```python
from build123d import *

# Parameters (mm, degrees)
F0_W      = 92
F0_H      = 42.9992415011
F0_W_2    = 39.8767858334
F0_H_2    = 7.2647114284
F0_W_3    = 8.2464283332
F0_H_3    = 15.8676442858
F1_DEPTH  = 2
F2_W      = 8.2464283332
F2_H      = 1.5
F3_DEPTH  = 17
F4_DEPTH  = 17
F6_DEPTH  = 2
F7_W      = 8
F7_H      = 3
F8_DEPTH  = 1
F10_W     = 8
F10_H     = 8
F11_DEPTH = 1
F9_W      = 8
F9_H      = 8
F12_DEPTH = 1
F13_W     = 8
F13_H     = 8
F14_DEPTH = 1
F15_W     = 8
F15_H     = 8
F16_DEPTH = 1
F17_W     = 92
F17_H     = 42.9992415011
F18_DEPTH = 15
F20_D     = 2
F20_DEPTH = 12
F20_TIP   = 0.600860619
F22_D     = 2
F22_DEPTH = 12
F22_TIP   = 0.600860619
F24_D     = 2
F24_DEPTH = 12
F24_TIP   = 0.600860619
F26_D     = 2
F26_DEPTH = 12
F26_TIP   = 0.600860619
F27_W     = 7.3435585946
F27_H     = 11.5889557712
F28_DEPTH = 3
F29_W     = 6.5705534071
F29_H     = 0.7730051875
F30_DEPTH = 0.3
F31_W     = 6.048291456
F31_H     = 0.9969957173
F32_DEPTH = 0.3
F33_R     = 5
F34_R     = 5
F35_R     = 5
F36_R     = 5
F37_W     = 120.588965714
F37_H     = 68.2177916169
F38_DEPTH = 0.6
F39_DEPTH = 25


with BuildPart() as f1:
    # F0 (on Top) → F1 (new body)
    with BuildSketch(Plane.XY):
        Rectangle(F0_W, F0_H)
        Polygon((-44, 3.6323557142), (-44, 19.5), (-4.1232141666, 19.5), (4.1232141666, 19.5), (44, 19.5), (44, 3.6323557142), (44, -3.6323557142), (44, -19.5), (4.1232141666, -19.5), (-4.1232141666, -19.5), (-44, -19.5), (-44, -3.6323557142), align=None, mode=Mode.SUBTRACT)
        with Locations((-24.0616070833, 0)):
            Rectangle(F0_W_2, F0_H_2)
        with Locations((24.0616070833, 0)):
            Rectangle(F0_W_2, F0_H_2)
        with Locations((0, -11.5661778571)):
            Rectangle(F0_W_3, F0_H_3)
        with Locations((0, 11.5661778571)):
            Rectangle(F0_W_3, F0_H_3)
        Rectangle(F0_W_3, F0_H_2)
    extrude(amount=F1_DEPTH)

    # F2 (on face) → F3 (join)
    with BuildSketch(Plane.XY.offset(2)):
        with Locations((0, 15.75)):
            Rectangle(F2_W, F2_H)
    extrude(amount=F3_DEPTH)

    # F2 (on face) → F4 (join)
    with BuildSketch(Plane.XY.offset(2)):
        with Locations((0, -15.75)):
            Rectangle(F2_W, F2_H)
    extrude(amount=F4_DEPTH)

    # F5 (on face) → F6 (join)
    with BuildSketch(Plane.XY.offset(2)):
        Polygon((-4.1232141666, -3.6323557142), (-4.1232141666, -15), (4.1232141666, -15), (4.1232141666, -3.6323557142), (4.1232141666, 3.6323557142), (4.1232141666, 15), (-4.1232141666, 15), (-4.1232141666, 3.6323557142), align=None)
    extrude(amount=F6_DEPTH)

    # F7 (on face) → F8 (join)
    with BuildSketch(Plane.XY.offset(19)):
        with Locations((0, -15)):
            Rectangle(F7_W, F7_H)
        with Locations((0, 15.0357708335)):
            Rectangle(F7_W, F7_H)
    extrude(amount=F8_DEPTH)

    # F10 (on Top) → F11 (join)
    with BuildSketch(Plane.XY):
        with Locations((-41.8757377899, 17.4122615717)):
            Rectangle(F10_W, F10_H)
    extrude(amount=F11_DEPTH)

    # F9 (on Top) → F12 (join)
    with BuildSketch(Plane.XY):
        with Locations((-42, -17.4996207505)):
            Rectangle(F9_W, F9_H)
    extrude(amount=F12_DEPTH)

    # F13 (on Top) → F14 (join)
    with BuildSketch(Plane.XY):
        with Locations((41.91535397, 17.2840473242)):
            Rectangle(F13_W, F13_H)
    extrude(amount=F14_DEPTH)

    # F15 (on Top) → F16 (join)
    with BuildSketch(Plane.XY):
        with Locations((41.8707623184, -17.4904118329)):
            Rectangle(F15_W, F15_H)
    extrude(amount=F16_DEPTH)

    # F17 (on face) → F18 (join)
    with BuildSketch(Plane.XY.offset(2)):
        Rectangle(F17_W, F17_H)
        Polygon((4.1232141666, -19.5), (-4.1232141666, -19.5), (-44, -19.5), (-44, -3.6323557142), (-44, 3.6323557142), (-44, 19.5), (-4.1232141666, 19.5), (4.1232141666, 19.5), (44, 19.5), (44, 3.6323557142), (44, -3.6323557142), (44, -19.5), align=None, mode=Mode.SUBTRACT)
    extrude(amount=F18_DEPTH)

    # F20
    with Locations(Plane.XY.offset(1)):
        with Locations((-41, -16.4998103753)):
            Hole(F20_D / 2, depth=F20_DEPTH)
            with Locations((0, 0, -(F20_DEPTH + F20_TIP / 2))):  # 118° drill point
                Cone(0, F20_D / 2, F20_TIP, mode=Mode.SUBTRACT)

    # F22
    with Locations(Plane.XY.offset(1)):
        with Locations((-40.937868895, 16.4561307859)):
            Hole(F22_D / 2, depth=F22_DEPTH)
            with Locations((0, 0, -(F22_DEPTH + F22_TIP / 2))):  # 118° drill point
                Cone(0, F22_D / 2, F22_TIP, mode=Mode.SUBTRACT)

    # F24
    with Locations(Plane.XY.offset(1)):
        with Locations((40.957676985, 16.3920236621)):
            Hole(F24_D / 2, depth=F24_DEPTH)
            with Locations((0, 0, -(F24_DEPTH + F24_TIP / 2))):  # 118° drill point
                Cone(0, F24_D / 2, F24_TIP, mode=Mode.SUBTRACT)

    # F26
    with Locations(Plane.XY.offset(1)):
        with Locations((40.9353811592, -16.4952059165)):
            Hole(F26_D / 2, depth=F26_DEPTH)
            with Locations((0, 0, -(F26_DEPTH + F26_TIP / 2))):  # 118° drill point
                Cone(0, F26_D / 2, F26_TIP, mode=Mode.SUBTRACT)

    # F27 (on face) → F28 (cut)
    with BuildSketch(Plane(origin=(-46, 0, 0), x_dir=(0, -1, 0), z_dir=(-1, 0, 0))):
        with Locations((-0.289877411, 11.2055221144)):
            Rectangle(F27_W, F27_H)
    extrude(amount=-F28_DEPTH, mode=Mode.SUBTRACT)

    # F29 (on face) → F30 (join)
    with BuildSketch(Plane.XZ.offset(21.4996207505)):
        with Locations((0, 12.4647244811)):
            Rectangle(F29_W, F29_H)
    extrude(amount=F30_DEPTH)

    # F31 (on face) → F32 (join)
    with BuildSketch(Plane(origin=(0, 21.4996207505, 0), x_dir=(-1, 0, 0), z_dir=(0, 1, 0))):
        with Locations((0, 13.2352923974)):
            Rectangle(F31_W, F31_H)
    extrude(amount=F32_DEPTH)

    # F33
    f33_edges = [f1.edges().sort_by_distance(p)[0] for p in [
        (-46, -21.499621, 8.5),
    ]]
    fillet(f33_edges, radius=F33_R)

    # F34
    f34_edges = [f1.edges().sort_by_distance(p)[0] for p in [
        (46, -21.499621, 8.5),
    ]]
    fillet(f34_edges, radius=F34_R)

    # F35
    f35_edges = [f1.edges().sort_by_distance(p)[0] for p in [
        (46, 21.499621, 8.5),
    ]]
    fillet(f35_edges, radius=F35_R)

    # F36
    f36_edges = [f1.edges().sort_by_distance(p)[0] for p in [
        (-46, 21.499621, 8.5),
    ]]
    fillet(f36_edges, radius=F36_R)

    # F37 (on Top) → F38 (join)
    with BuildSketch(Plane.XY):
        Rectangle(F37_W, F37_H)
    extrude(amount=F38_DEPTH)

    # F39 (cut): faces of the model
    f39_faces = [f1.faces().sort_by_distance(p)[0] for p in [
        (-23.0397011823, -11.2685281209, 0.6),
        (-23.0049653202, 11.2600123957, 0.6),
        (22.9874600432, 11.2593805949, 0.6),
        (23.0186221767, -11.261509687, 0.6),
    ]]
    extrude(f39_faces, amount=-F39_DEPTH, mode=Mode.SUBTRACT)


solid = f1.part
```
Input: part model. Units: mm. Frame: model coordinates. A direction names the side the tool comes from. Round coordinates to 2 decimals unless told otherwise and drop trailing zeros. Order: outer loops, then holes, each group sorted by start corner. A loop starts at its lowest first (then second) coordinate and runs counter-clockwise, first axis right, second up. Notation, with made-up numbers: (89.25, -37.75) - (102.25, -37.75) arc R21 ccw to (102.25, -3.75) - close; hole circle Ø3 at (0, 0). An arc over 180 degrees is marked (long way). Answer in a Markdown table with one row per item.
Item 1: Reachability of faces 1 (the cylindrical face through (-44.5, 20.07, 8.69)), 2 (the cylindrical face through (44.5, -20.07, 8.91)), 3 (the flat face through (0, -16.5, 11)), 4 (the flat face through (0, 15, 11)), 5 (the cylindrical face through (44.57, 20, 8.69)) from +Z, -Z, +X, -X, +Y, -Y: full face, straight path, thin tool, end or side. Return the list, or none.
Model answer:
| item | result |
|---|---|
| face 1 | +Z, -X, +Y |
| face 2 | +Z, +X, -Y |
| face 3 | +Z |
| face 4 | none |
| face 5 | +Z, +X, +Y |
Item 2: Section query B-B (x = 8). Return the cut outline in (y, z).
Model answer:
| item | result |
|---|---|
| outline | (-34.11, 0) - (-19.5, 0) - (-19.5, 17) - (-21.5, 17) - (-21.5, 0.6) - (-34.11, 0.6) - close; (-3.63, 0) - (3.63, 0) - (3.63, 2) - (-3.63, 2) - close; (19.5, 0) - (34.11, 0) - (34.11, 0.6) - (21.5, 0.6) - (21.5, 17) - (19.5, 17) - close |
Item 3: Mould query, pull axis Z, two halves, no side actions, for faces 6 (the flat face through (0, -15, 11)), 7 (the flat face through (41, -15, 1)), 8 (the flat face through (-4.123, 0, 3)). Classes: released by +Z, released by -Z, zero draft, split by the parting line, or undercut.
Model answer:
| item | result |
|---|---|
| face 6 | undercut |
| face 7 | released by +Z |
| face 8 | zero draft |
Item 4: Pin query (flat end, axial travel): pin 1 (6 mm diameter, centred on y = 24, z = 11.5, fed in from +X); pin 2 (8 mm diameter, centred on y = 7.5, z = 17.5, fed in from +X); pin 3 (1.5 mm diameter, centred on x = -44.5, y = 6, fed in from +Z). Return the tip coordinate at first contact, or that it passes through.
Model answer:
| item | result |
|---|---|
| pin 1 | stops at x = 43.18 |
| pin 2 | stops at x = 46 |
| pin 3 | stops at z = 17 |
Item 5: Section query A-A (z = 15.25). Return the cut outline in (x, y), then the cut area to 3 significant figures.
Model answer:
| item | result |
|---|---|
| outline | (-46, -16.5) arc R5 ccw to (-41, -21.5) - (41, -21.5) arc R5 ccw to (46, -16.5) - (46, 16.5) arc R5 ccw to (41, 21.5) - (-41, 21.5) arc R5 ccw to (-46, 16.5) - (-46, 3.96) - (-44, 3.96) - (-44, 19.5) - (44, 19.5) - (44, -19.5) - (-44, -19.5) - (-44, -3.38) - (-46, -3.38) - close; (-4.12, -16.5) - (4.12, -16.5) - (4.12, -15) - (-4.12, -15) - close; (-4.12, 15) - (4.12, 15) - (4.12, 16.5) - (-4.12, 16.5) - close |
| area | 513 mm² |
Item 6: Line query: line 1 (X direction, y = -16, z = 14.5); line 2 (Y direction, x = 1.5, z = 9.5); line 3 (Y direction, x = -41, z = 0.8). Output: solid intervals per line, ascending.
Model answer:
| item | result |
|---|---|
| line 1 | x = -46 to -44, -4.12 to 4.12, 44 to 46 |
| line 2 | y = -21.5 to -19.5, -16.5 to -15, 15 to 16.5, 19.5 to 21.5 |
| line 3 | y = -21.5 to -17.5, -15.5 to -13.5, -3.63 to 3.63, 13.41 to 15.46, 17.45 to 21.5 |
